Check sheet for the modelled part. Datum: model origin and axes. Units: mm. A direction names the side the tool comes from. Give positions to 0.01 mm unless a question says otherwise; leave off trailing zeros. Write each loop counter-clockwise with the first axis right and the second up, starting at its lowest first coordinate (ties: lowest second). Pieces come first, ordered by that corner, then holes. Notation, with made-up numbers: M 81.5,-26.5 L 110.5,-26.5 A22 cw 110.5,-14.5 Z; hole C 9,14.5 d4. An arc over 180 degrees is marked long. Use CSV: the item, a comma, the result in double quotes. Start each with the question number.
1. Mould release check, pull along X, two halves, no side actions. Record for faces 5 (the face through (-37.788, 5.102, 1.602)), 6 (the face through (-8, 5, 5)), 7 (the face through (-3.666, 0.377, 2.465)), 8 (the face through (-41.774, 9.62, 2.465)): +X half, -X half, draft (parallel to the pull), parting line (faces both ways), or undercut.
2. Access from +Z, -Z, +X, -X, +Y, -Y to the whole of each face (thin tool, end or side, straight path). Record for faces 1 (the face through (-35, 5, 5)), 2 (the face through (-44.836, 5.086, 2.465)), 3 (the face through (-35, 10, 2)), 4 (the face through (-10, 10, 2)).
3. Cross-section at B-B, the plane x = -35. Enter the section's corners in (y, z).
4. Scan lines: line 1 (X direction, y = 17, z = 6.25); line 2 (Y direction, x = -9, z = 1.25); line 3 (Z direction, x = -6.5, y = 6.5). Record each from-to range of solid material in increasing order.
5. Cross-section at A-A, the plane z = 2.25. Enter the section's corners in (x, y), and give its area (3 significant figures).
6. Depth check by flat-ended pin: P1, Ø3, axis at x = -11, y = 5, coming from the +Z side; P2, Ø4.5, axis at x = -39.44, y = 5.03, coming from the +Z side; P3, Ø2, axis at y = 10.5, z = 6, coming from the +X side. Enter the tip coordinate at first touch or a pass-through.
7. Cross-section at D-D, the plane z = 4.5. Enter the section's corners in (x, y), and give its area (3 significant figures).
8. Cross-section at C-C, the plane y = 16.75. Enter the section's corners in (x, z), and give its area (3 significant figures).
from build123d import *

# Parameters (mm, degrees)
F0_R           = 1.7
F1_DEPTH       = 5
F2_DEPTH       = 15
F4_D           = 3.3
F4_CSINK_D     = 6.8
F4_CSINK_ANGLE = 90


with BuildPart() as f1:
    # F0 (on Top) → F1 (new body)
    with BuildSketch(Plane.XY):
        with BuildLine():
            Line((-39.4, 0), (-30.654659, 0))
            Line((-30.654659, 0), (-30.654659, 10))
            Line((-30.654659, 10), (-39.386656, 10))
            Line((-39.386656, 10), (-40.009414, 10))
            ThreePointArc((-40.009414, 10), (-41.798277, 9.611144), (-43.374257, 8.679732))
            ThreePointArc((-43.374257, 8.679732), (-44.836341, 5.029774), (-43.374257, 1.379816))
            ThreePointArc((-43.374257, 1.379816), (-41.689998, 0.386223), (-39.773025, 0))
            Line((-39.773025, 0), (-39.4, 0))
        make_face()
        with Locations((-39.4, 5)):
            Circle(F0_R, mode=Mode.SUBTRACT)
        Polygon((-30.654659, 0), (-14.532625, 0), (-14.532625, 10), (-14.532625, 18), (-30.654659, 18), (-30.654659, 10), align=None)
        with BuildLine():
            Line((-6, 0), (-5.471228, 0))
            ThreePointArc((-5.471228, 0), (-3.641152, 0.386148), (-2.029729, 1.335675))
            ThreePointArc((-2.029729, 1.335675), (-0.646469, 4.881091), (-2.029729, 8.426508))
            ThreePointArc((-2.029729, 8.426508), (-3.879298, 9.555319), (-6, 10))
            Line((-6, 10), (-14.532625, 10))
            Line((-14.532625, 10), (-14.532625, 0))
            Line((-14.532625, 0), (-6, 0))
        make_face()
        with Locations((-6, 5)):
            Circle(F0_R, mode=Mode.SUBTRACT)
        with Locations((-39.4, 5)):
            Circle(F0_R)
        with Locations((-6, 5)):
            Circle(F0_R)
    extrude(amount=F1_DEPTH)

    # F0 (on Top) → F2 (join)
    with BuildSketch(Plane.XY):
        Polygon((-30.654659, 0), (-14.532625, 0), (-14.532625, 10), (-14.532625, 18), (-30.654659, 18), (-30.654659, 10), align=None)
    extrude(amount=F2_DEPTH)

    # F4 (through all)
    with Locations(Plane.XY.offset(5)):
        with Locations((-39.436341, 5.029774)):
            CounterSinkHole(F4_D / 2, F4_CSINK_D / 2, counter_sink_angle=F4_CSINK_ANGLE)


solid = f1.part
Worked answers:
1,face 5,"undercut"
1,face 6,"draft"
1,face 7,"+X half"
1,face 8,"-X half"
2,face 1,"+Z, -X, +Y, -Y"
2,face 2,"+Z, -Z, -X"
2,face 3,"+Z, -Z, -X, +Y"
2,face 4,"+Z, -Z, +X, +Y"
3,outline,"M 0,0 L 10,0 L 10,5 L 0,5 Z"
4,line 1,"x = -30.65 to -14.53"
4,line 2,"y = 0 to 10"
4,line 3,"z = 0 to 5"
5,outline,"M -43.37,1.38 A5.88 ccw -39.77,0 L -5.47,0 A5.79 ccw -2.03,1.34 A5.24 ccw -2.03,8.43 A6.38 ccw -6,10 L -14.53,10 L -14.53,18 L -30.65,18 L -30.65,10 L -40.01,10 A5.75 ccw -43.37,8.68 A5.29 ccw Z; hole C -39.44,5.03 d3.3"
5,area,"541 mm^2"
6,P1,"stops at z = 5"
6,P2,"stops at z = 3.85"
6,P3,"stops at x = -14.53"
7,outline,"M -43.37,1.38 A5.88 ccw -39.77,0 L -5.47,0 A5.79 ccw -2.03,1.34 A5.24 ccw -2.03,8.43 A6.38 ccw -6,10 L -14.53,10 L -14.53,18 L -30.65,18 L -30.65,10 L -40.01,10 A5.75 ccw -43.37,8.68 A5.29 ccw Z; hole C -39.44,5.03 d5.8"
7,area,"523 mm^2"
8,outline,"M -30.65,0 L -14.53,0 L -14.53,15 L -30.65,15 Z"
8,area,"242 mm^2"
